Can you work these out from the model? Positions are in its coordinate system, mm. Give positions to 0.01 mm unless a question says otherwise; leave off trailing zeros. Write each loop counter-clockwise with the first axis right and the second up, starting at its lowest first coordinate (ties: lowest second). Pieces come first, ordered by that corner, then holes. Notation, with made-up numbers: (12.25, 15.25) -> (67.25, 15.25) arc R25 ccw to (67.25, 53.25) -> close; hole circle Ø3 at (-36, 70). An arc over 180 degrees is marked (long way). Answer as CSV lines item,"result". Start each with the question number.
1. If we section it at C-C on z = 1.35: Count the separate pieces of the cut face and the enclosed holes in it, plus the area to 3 significant figures.
2. If we section it at A-A on x = 97: Write out the boundary of the cut face in (y, z), plus the area to 3 significant figures.
3. I need wall thicknesses on line 1 (Y direction, x = 102.5, z = 2); line 2 (X direction, y = 156, z = 1.1); line 3 (X direction, y = 83, z = 2.3). Which ranges of each line are inside material? Lowest first, please. Write a range as [from, to].
4. If we section it at B-B on x = 55.75: Write out the boundary of the cut face in (y, z), plus the area to 4 significant figures.
Autodesk Inventor part; units mm, degrees
ref_plane "YZ Plane" through (0, 0, 0) normal (1, 0, 0) x (0, 1, 0)
ref_plane "XZ Plane" through (0, 0, 0) normal (0, 1, 0) x (-1, 0, 0)
ref_plane "XY Plane" through (0, 0, 0) normal (0, 0, 1) x (1, 0, 0)
sketch "Sketch1" plane through (0, 0, 0) normal (0, 0, 1) x (1, 0, 0)
  line L0 (-3, 166.036) -> (167, 166.036)
  line L1 (177, 156.036) -> (177, 11.036)
  line L2 (167, 1.036) -> (-3, 1.036)
  line L3 (-13, 11.036) -> (-13, 156.036)
  arc A0 (177, 156.036) -> (167, 166.036) centre (167, 156.036) ccw
  arc A1 (-3, 166.036) -> (-13, 156.036) centre (-3, 156.036) ccw
  arc A2 (-13, 11.036) -> (-3, 1.036) centre (-3, 11.036) ccw
  arc A3 (167, 1.036) -> (177, 11.036) centre (167, 11.036) ccw
  circle A4 centre (26.45, 119.036) radius 22
  circle A5 centre (137.55, 119.036) radius 22
  line L4 (59.95, 132.136) -> (62.7, 132.136)
  line L5 (63.2, 131.636) -> (63.2, 106.436)
  line L6 (62.7, 105.936) -> (59.95, 105.936)
  line L7 (59.45, 106.436) -> (59.45, 131.636)
  line L8 (101.3, 132.136) -> (104.05, 132.136)
  line L9 (104.55, 131.636) -> (104.55, 106.436)
  line L10 (104.05, 105.936) -> (101.3, 105.936)
  line L11 (100.8, 106.436) -> (100.8, 131.636)
  line L12 (13.85, 86.036) -> (39.05, 86.036)
  line L13 (39.55, 85.536) -> (39.55, 82.786)
  line L14 (39.05, 82.286) -> (13.85, 82.286)
  line L15 (13.35, 82.786) -> (13.35, 85.536)
  line L16 (124.95, 86.036) -> (150.15, 86.036)
  line L17 (150.65, 85.536) -> (150.65, 82.786)
  line L18 (150.15, 82.286) -> (124.95, 82.286)
  line L19 (124.45, 82.786) -> (124.45, 85.536)
  line L20 (26.45, 119.036) -> (137.55, 119.036) construction
  arc A6 (59.95, 132.136) -> (59.45, 131.636) centre (59.95, 131.636) ccw
  arc A7 (63.2, 131.636) -> (62.7, 132.136) centre (62.7, 131.636) ccw
  arc A8 (62.7, 105.936) -> (63.2, 106.436) centre (62.7, 106.436) ccw
  arc A9 (59.45, 106.436) -> (59.95, 105.936) centre (59.95, 106.436) ccw
  arc A10 (100.8, 106.436) -> (101.3, 105.936) centre (101.3, 106.436) ccw
  arc A11 (104.05, 105.936) -> (104.55, 106.436) centre (104.05, 106.436) ccw
  arc A12 (101.3, 132.136) -> (100.8, 131.636) centre (101.3, 131.636) ccw
  arc A13 (104.55, 131.636) -> (104.05, 132.136) centre (104.05, 131.636) ccw
  arc A14 (39.55, 85.536) -> (39.05, 86.036) centre (39.05, 85.536) ccw
  arc A15 (39.05, 82.286) -> (39.55, 82.786) centre (39.05, 82.786) ccw
  arc A16 (13.35, 82.786) -> (13.85, 82.286) centre (13.85, 82.786) ccw
  arc A17 (13.85, 86.036) -> (13.35, 85.536) centre (13.85, 85.536) ccw
  circle A18 centre (49.55, 142.286) radius 1.5
  circle A19 centre (3.35, 142.286) radius 1.5
  circle A20 centre (49.55, 95.786) radius 1.5
  circle A21 centre (2.35, 95.786) radius 1.5
  line L21 (49.55, 142.286) -> (49.55, 95.786) construction
  line L22 (49.55, 142.286) -> (3.35, 142.286) construction
  arc A22 (124.95, 86.036) -> (124.45, 85.536) centre (124.95, 85.536) ccw
  arc A23 (124.45, 82.786) -> (124.95, 82.286) centre (124.95, 82.786) ccw
  arc A24 (150.15, 82.286) -> (150.65, 82.786) centre (150.15, 82.786) ccw
  arc A25 (150.65, 85.536) -> (150.15, 86.036) centre (150.15, 85.536) ccw
  circle A26 centre (114.45, 142.286) radius 1.5
  circle A27 centre (160.65, 142.286) radius 1.5
  circle A28 centre (160.65, 95.786) radius 1.5
  circle A29 centre (114.45, 95.786) radius 1.5
  line L23 (160.65, 142.286) -> (160.65, 95.786) construction
  line L24 (114.45, 142.286) -> (160.65, 142.286) construction
  line L25 (8, 59.036) -> (104, 59.036)
  line L26 (105, 58.036) -> (105, 20.036)
  line L27 (104, 19.036) -> (8, 19.036)
  line L28 (7, 20.036) -> (7, 58.036)
  arc A30 (8, 59.036) -> (7, 58.036) centre (8, 58.036) ccw
  arc A31 (7, 20.036) -> (8, 19.036) centre (8, 20.036) ccw
  arc A32 (104, 19.036) -> (105, 20.036) centre (104, 20.036) ccw
  arc A33 (105, 58.036) -> (104, 59.036) centre (104, 58.036) ccw
  circle A34 centre (55.75, 75.336) radius 3.25
  circle A35 centre (73.25, 75.336) radius 3.25
  circle A36 centre (90.75, 75.336) radius 3.25
  circle A37 centre (108.25, 75.336) radius 3.25
  line L29 (73.25, 75.336) -> (90.75, 75.336) construction
  line L30 (39.55, 82.286) -> (124.45, 82.286) construction
  circle A38 centre (113, 50.036) radius 3.075
  circle A39 centre (113, 28.036) radius 3.075
  line L31 (113, 50.036) -> (113, 28.036) construction
  circle A40 centre (137, 50.036) radius 1.85
  circle A41 centre (126, 39.036) radius 1.85
  circle A42 centre (137, 39.036) radius 1.85
  circle A43 centre (137, 28.036) radius 1.85
  circle A44 centre (148, 39.036) radius 1.85
  circle A45 centre (163, 39.036) radius 3.25
  circle A46 centre (167, 156.036) radius 1.5
  circle A47 centre (-3, 156.036) radius 1.5
  circle A48 centre (167, 11.036) radius 1.5
  circle A49 centre (-3, 11.036) radius 1.5
  circle A50 centre (9.5, 67.036) radius 1.5
  circle A51 centre (102.5, 67.036) radius 1.5
  circle A52 centre (9.5, 11.036) radius 1.5
  circle A53 centre (102.5, 11.036) radius 1.5
  point P0 (0, 0)
  point P1 (-13, 166.036)
  point P2 (177, 1.036)
  point P3 (-13, 1.036)
  point P4 (59.45, 132.136)
  point P5 (63.2, 105.936)
  point P6 (63.2, 132.136)
  point P7 (100.8, 132.136)
  point P8 (104.55, 105.936)
  point P9 (104.55, 132.136)
  point P10 (13.35, 86.036)
  point P11 (13.35, 82.286)
  point P12 (124.45, 86.036)
  point P13 (150.65, 82.286)
  point P14 (104.55, 119.036)
  point P15 (63.2, 119.036)
  point P16 (26.45, 86.036)
  point P17 (137.55, 86.036)
  point P18 (26.45, 142.286)
  point P19 (49.55, 119.036)
  point P20 (160.65, 119.036)
  point P21 (137.55, 142.286)
  point P22 (105, 19.036)
  point P23 (105, 59.036)
  point P24 (7, 19.036)
  point P25 (82, 75.336)
  point P26 (82, 82.286)
  point P27 (113, 39.036)
  point P28 (105, 39.036)
  dimension "d0" = 190
  dimension "d1" = 165
  dimension "d2" = 10
  dimension "d3" = 44
  dimension "d4" = 44
  dimension "d5" = 111.1
  dimension "d6" = 39.45
  dimension "d7" = 39.45
  dimension "d8" = 47
  dimension "d9" = 3.75
  dimension "d10" = 26.2
  dimension "d11" = 3.75
  dimension "d12" = 26.2
  dimension "d13" = 3.75
  dimension "d14" = 26.2
  dimension "d15" = 3.75
  dimension "d16" = 26.2
  dimension "d17" = 33
  dimension "d18" = 33
  dimension "d19" = 33
  dimension "d20" = 33
  dimension "d21" = 0.5
  dimension "a" = 3
  dimension "d23" = 3
  dimension "d24" = 3
  dimension "d25" = 3
  dimension "d26" = 46.2
  dimension "d27" = 47.2
  dimension "d28" = 46.5
  dimension "d29" = 0.5
  dimension "d30" = 3
  dimension "d31" = 3
  dimension "d32" = 3
  dimension "d33" = 3
  dimension "d34" = 46.2
  dimension "d35" = 46.5
  dimension "d36" = 98
  dimension "d37" = 40
  dimension "d38" = 20
  dimension "d39" = 18
  dimension "d40" = 1
  dimension "d41" = 23.25
  dimension "b" = 6.5
  dimension "d43" = 6.5
  dimension "d44" = 6.5
  dimension "d45" = 6.5
  dimension "d" = 17.5
  dimension "d47" = 17.5
  dimension "d48" = 17.5
  dimension "d49" = 16.3
  dimension "e" = 6.15
  dimension "d51" = 6.15
  dimension "d52" = 22
  dimension "d53" = 8
  dimension "i" = 3.7
  dimension "d55" = 3.7
  dimension "d56" = 3.7
  dimension "d57" = 3.7
  dimension "d58" = 3.7
  dimension "d59" = 22
  dimension "d60" = 11
  dimension "d61" = 22
  dimension "d62" = 11
  dimension "d68" = 6.5
extrude "Extrusion1" add sketch "Sketch1" along normal blind 3 contours L0 A0 L1 A3 L2 A2 L3 A1 | A50 | A51 | A52 | A53
extrude "Extrusion2" cut sketch "Sketch1" along normal blind 3 contours A50 | A51 | A52 | A53
equation "\"d23\" = a"
equation "\"d24\" = a"
equation "\"d25\" = a"
equation "\"d30\" = a"
equation "\"d31\" = a"
equation "\"d32\" = a"
equation "\"d33\" = a"
equation "\"d43\" = b"
equation "\"d44\" = b"
equation "\"d45\" = b"
properties part number "Front"
Computed values:
1,separate pieces,"1"
1,enclosed holes,"35"
1,area,"23,500 mm2"
2,outline,"(1.04, 0) -> (19.04, 0) -> (19.04, 3) -> (1.04, 3) -> close; (59.04, 0) -> (166.04, 0) -> (166.04, 3) -> (59.04, 3) -> close"
2,area,"375 mm2"
3,line 1,"y = [1.04, 9.54], [12.54, 19.04], [59.04, 65.54], [68.54, 105.94], [132.14, 166.04]"
3,line 2,"x = [-13, -4.5], [-1.5, 165.5], [168.5, 177]"
3,line 3,"x = [-13, 13.35], [39.55, 124.45], [150.65, 177]"
4,outline,"(1.04, 0) -> (19.04, 0) -> (19.04, 3) -> (1.04, 3) -> close; (59.04, 0) -> (72.09, 0) -> (72.09, 3) -> (59.04, 3) -> close; (78.59, 0) -> (166.04, 0) -> (166.04, 3) -> (78.59, 3) -> close"
4,area,"355.5 mm2"
